Can you work these out from the model? Positions are in its coordinate system, mm. Face numbers are marked on the shaded views. A direction names the side the tool comes from. Round coordinates to 2 decimals unless told otherwise and drop trailing zeros. Loops run counter-clockwise (first coordinate to the right, second up) from the corner with the lowest first, then second, coordinate; pieces in that order, holes last. Notation, with made-up numbers: M -3,66 L 26,66 A9 ccw 26,79 Z; hole C 86.5,40 d7. An arc over 180 degrees is marked long. Use a Markdown table: item, result. Add a question column.
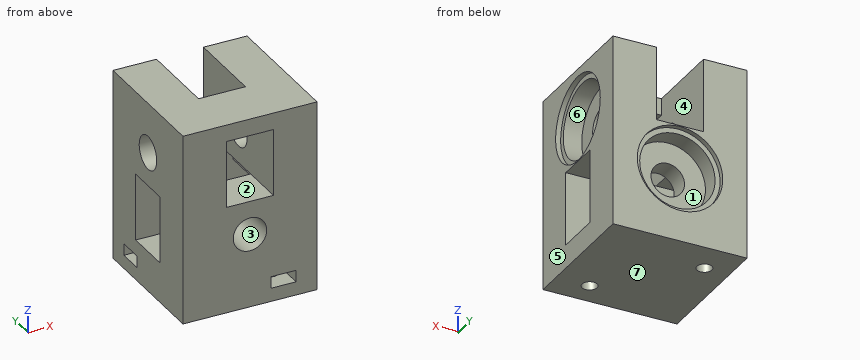
```python
from build123d import *

# Parameters (mm, degrees)
ESQUISSE1_W              = 40
ESQUISSE1_H              = 40
BOSS_EXTRU_1_DEPTH       = 50
ESQUISSE2_R              = 5
ENL_V_MAT_EXTRU_1_DEPTH  = 41
ESQUISSE3_R              = 5
ENL_V_MAT_EXTRU_2_DEPTH  = 41
ESQUISSE4_W              = 20
ESQUISSE4_H              = 14
ENL_V_MAT_EXTRU_3_DEPTH  = 29
ESQUISSE5_W              = 14
ESQUISSE5_H              = 20
ENL_V_MAT_EXTRU_4_DEPTH  = 29
ESQUISSE6_W              = 22
ESQUISSE6_H              = 14
ENL_V_MAT_EXTRU_5_DEPTH  = 24
ESQUISSE7_W              = 14
ESQUISSE7_H              = 22
ENL_V_MAT_EXTRU_6_DEPTH  = 24
ESQUISSE8_R              = 11.25
ENL_V_MAT_EXTRU_7_DEPTH  = 7
ESQUISSE9_R              = 12.75
ENL_V_MAT_EXTRU_8_DEPTH  = 1.5
ESQUISSE10_R             = 11.25
ENL_V_MAT_EXTRU_9_DEPTH  = 7
ESQUISSE11_R             = 12.75
ENL_V_MAT_EXTRU_10_DEPTH = 1.5
ESQUISSE12_W             = 40
ESQUISSE12_H             = 40
BOSS_EXTRU_2_DEPTH       = 7
ESQUISSE13_R             = 2.25
ENL_V_MAT_EXTRU_11_DEPTH = 15
ESQUISSE14_W             = 3.5
ESQUISSE14_H             = 7.5
ENL_V_MAT_EXTRU_12_DEPTH = 12
ESQUISSE15_W             = 7.5
ESQUISSE15_H             = 3.5
ENL_V_MAT_EXTRU_13_DEPTH = 12


with BuildPart() as part:
    # Esquisse1 → Boss.-Extru.1 (new body)
    with BuildSketch(Plane.XY):
        with Locations((-20, 20)):
            Rectangle(ESQUISSE1_W, ESQUISSE1_H)
    extrude(amount=BOSS_EXTRU_1_DEPTH)

    # Esquisse2 → Enlèv. mat.-Extru.1 (cut, through all)
    with BuildSketch(Plane(origin=(0, 40, 0), x_dir=(1, 0, 0), z_dir=(0, 1, 0))):
        with Locations(Location((-20, -15, 0), (0, 0, 270))):  # turned: the seam where the file's is
            Circle(ESQUISSE2_R)
    extrude(amount=-ENL_V_MAT_EXTRU_1_DEPTH, mode=Mode.SUBTRACT)

    # Esquisse3 → Enlèv. mat.-Extru.2 (cut, through all)
    with BuildSketch(Plane.ZY.offset(40)):
        with Locations((35, 20)):
            Circle(ESQUISSE3_R)
    extrude(amount=-ENL_V_MAT_EXTRU_2_DEPTH, mode=Mode.SUBTRACT)

    # Esquisse4 → Enlèv. mat.-Extru.3 (cut)
    with BuildSketch(Plane.ZY.offset(40)):
        with Locations((15, 20)):
            Rectangle(ESQUISSE4_W, ESQUISSE4_H)
    extrude(amount=-ENL_V_MAT_EXTRU_3_DEPTH, mode=Mode.SUBTRACT)

    # Esquisse5 → Enlèv. mat.-Extru.4 (cut)
    with BuildSketch(Plane.XZ):
        with Locations((-20, 35)):
            Rectangle(ESQUISSE5_W, ESQUISSE5_H)
    extrude(amount=-ENL_V_MAT_EXTRU_4_DEPTH, mode=Mode.SUBTRACT)

    # Esquisse6 → Enlèv. mat.-Extru.5 (cut)
    with BuildSketch(Plane(origin=(0, 0, 0), x_dir=(0, 0, -1), z_dir=(1, 0, 0))):
        with Locations((-11, 20)):
            Rectangle(ESQUISSE6_W, ESQUISSE6_H)
    extrude(amount=-ENL_V_MAT_EXTRU_5_DEPTH, mode=Mode.SUBTRACT)

    # Esquisse7 → Enlèv. mat.-Extru.6 (cut)
    with BuildSketch(Plane(origin=(0, 40, 0), x_dir=(1, 0, 0), z_dir=(0, 1, 0))):
        with Locations((-20, -39)):
            Rectangle(ESQUISSE7_W, ESQUISSE7_H)
    extrude(amount=-ENL_V_MAT_EXTRU_6_DEPTH, mode=Mode.SUBTRACT)

    # Esquisse8 → Enlèv. mat.-Extru.7 (cut)
    with BuildSketch(Plane(origin=(0, 0, 0), x_dir=(0, 0, -1), z_dir=(1, 0, 0))):
        with Locations(Location((-35, 20, 0), (0, 0, 90))):  # turned: the seam where the file's is
            Circle(ESQUISSE8_R)
    extrude(amount=-ENL_V_MAT_EXTRU_7_DEPTH, mode=Mode.SUBTRACT)

    # Esquisse9 → Enlèv. mat.-Extru.8 (cut)
    with BuildSketch(Plane(origin=(0, 0, 0), x_dir=(0, 0, -1), z_dir=(1, 0, 0))):
        with Locations(Location((-35, 20, 0), (0, 0, 90))):  # turned: the seam where the file's is
            Circle(ESQUISSE9_R)
    extrude(amount=-ENL_V_MAT_EXTRU_8_DEPTH, mode=Mode.SUBTRACT)

    # Esquisse10 → Enlèv. mat.-Extru.9 (cut)
    with BuildSketch(Plane(origin=(0, 40, 0), x_dir=(1, 0, 0), z_dir=(0, 1, 0))):
        with Locations(Location((-20, -15, 0), (0, 0, 270))):  # turned: the seam where the file's is
            Circle(ESQUISSE10_R)
    extrude(amount=-ENL_V_MAT_EXTRU_9_DEPTH, mode=Mode.SUBTRACT)

    # Esquisse11 → Enlèv. mat.-Extru.10 (cut)
    with BuildSketch(Plane(origin=(0, 40, 0), x_dir=(1, 0, 0), z_dir=(0, 1, 0))):
        with Locations(Location((-20, -15, 0), (0, 0, 270))):  # turned: the seam where the file's is
            Circle(ESQUISSE11_R)
    extrude(amount=-ENL_V_MAT_EXTRU_10_DEPTH, mode=Mode.SUBTRACT)

    # Esquisse12 → Boss.-Extru.2 (add)
    with BuildSketch(Plane(origin=(0, 0, 0), x_dir=(-1, 0, 0), z_dir=(0, 0, -1))):
        with Locations((20, 20)):
            Rectangle(ESQUISSE12_W, ESQUISSE12_H)
    extrude(amount=BOSS_EXTRU_2_DEPTH)

    # Esquisse13 → Enlèv. mat.-Extru.11 (cut)
    with BuildSketch(Plane(origin=(0, 0, -7), x_dir=(-1, 0, 0), z_dir=(0, 0, -1))):
        with Locations((10, 7.5)):
            Circle(ESQUISSE13_R)
        with Locations((32.5, 30)):
            Circle(ESQUISSE13_R)
    extrude(amount=-ENL_V_MAT_EXTRU_11_DEPTH, mode=Mode.SUBTRACT)

    # Esquisse14 → Enlèv. mat.-Extru.12 (cut)
    with BuildSketch(Plane.ZY.offset(40)):
        with Locations((-1.25, 30)):
            Rectangle(ESQUISSE14_W, ESQUISSE14_H)
    extrude(amount=-ENL_V_MAT_EXTRU_12_DEPTH, mode=Mode.SUBTRACT)

    # Esquisse15 → Enlèv. mat.-Extru.13 (cut)
    with BuildSketch(Plane.XZ):
        with Locations((-10, -1.25)):
            Rectangle(ESQUISSE15_W, ESQUISSE15_H)
    extrude(amount=-ENL_V_MAT_EXTRU_13_DEPTH, mode=Mode.SUBTRACT)


solid = part.part
```
(1) Thinking about a two-plate mould opening in Z: for the marked faces 4, 5, 6 and 7, which applies, released by +Z, released by -Z, zero draft, split by the parting line, or undercut?
(2) If I drill on probe 1 along Z at (x, y) = (-20, 10.25); probe 2 along Y at (x, z) = (-10, -5); probe 3 along X at (y, z) = (39.25, 15), over which ranges is the centre line in solid material (lowest first)? Write a range as [from, to].
(3) Suppose I cut it at B-B on x = -20. Count the separate pieces of the cut face and the enclosed holes in it, and give its area (3 significant figures).
(4) On a 3-axis mill with a long thin cutter (end or side, diameter ignored), from which of +Z, -Z, +X, -X, +Y, -Y can I reach the whole of each face in a straight line? I mean the marked faces 1, 2 and 3. Say none if no direction works.
(5) Suppose I cut it at A-A on z = 15. List the corners of the cut face in (x, y) for me, and give its area (3 significant figures).
(6) Suppose I cut it at C-C on x = -36. List the corners of the cut face in (y, z) for me.
(7) I'm going to push flat-ended pins straight in: pin 1 (4 mm diameter, centred on x = -15.5, z = 34, fed in from -Y); pin 2 (10 mm diameter, centred on x = -23.5, z = 22.5, fed in from -Y); pin 3 (2.5 mm diameter, centred on x = -10, y = 7.5, fed in from -Z); pin 4 (23 mm diameter, centred on y = 20, z = 35, fed in from +X). Where does each tip first touch, or does it pass through?
Results below:
| question | item | result |
|---|---|---|
| 1 | face 4 | undercut |
| 1 | face 5 | zero draft |
| 1 | face 6 | undercut |
| 1 | face 7 | released by -Z |
| 2 | probe 1 | z = [-7, 10], [20, 25], [45, 50] |
| 2 | probe 2 | y = [0, 5.25], [9.75, 40] |
| 2 | probe 3 | x = [-40, -32.75], [-7.25, 0] |
| 3 | separate pieces | 4 |
| 3 | enclosed holes | 0 |
| 3 | area | 691 mm² |
| 4 | face 1 | +Y |
| 4 | face 2 | -Y |
| 4 | face 3 | +Y, -Y |
| 5 | outline | M -40,0 L -25,0 L -25,13 L -40,13 Z; M -40,27 L -25,27 L -25,33 L -31.25,33 L -31.25,38.5 L -32.75,38.5 L -32.75,40 L -40,40 Z; M -15,0 L 0,0 L 0,13 L -15,13 Z; M -15,27 L 0,27 L 0,40 L -7.25,40 L -7.25,38.5 L -8.75,38.5 L -8.75,33 L -15,33 Z |
| 5 | area | 688 mm² |
| 6 | outline | M 0,-7 L 40,-7 L 40,50 L 0,50 Z; hole M 13,5 L 27,5 L 27,25 L 13,25 Z; hole C 20,35 d10; hole M 26.25,-3 L 33.75,-3 L 33.75,0.5 L 26.25,0.5 Z |
| 7 | pin 1 | passes through |
| 7 | pin 2 | stops at y = 0 |
| 7 | pin 3 | stops at z = 8 |
| 7 | pin 4 | stops at x = -1.5 |
